CAD build for the part. Positions are in the model's coordinates, mm. A direction names the side the tool comes from. Coordinates: 2 decimals unless noted, no trailing zeros. Loops run counter-clockwise (first coordinate to the right, second up) from the corner with the lowest first, then second, coordinate; pieces in that order, holes last. Notation, with made-up numbers: (15.25, 20) -> (40.25, 20) arc R26 cw to (40.25, 48) -> close; hole circle Ø8 at (65, 57). An arc over 180 degrees is marked (long way). Write each question's results on one line, items separated by ' | '.
from build123d import *

# Parameters (mm, degrees)
SKETCH1_R           = 4
SKETCH1_R_2         = 1.625
BOSS_EXTRUDE2_DEPTH = 20
SKETCH2_R           = 4.9
BOSS_EXTRUDE3_DEPTH = 62
SKETCH6_R           = 1.625
CUT_EXTRUDE3_DEPTH  = 20


with BuildPart() as part:
    # Sketch1 → Boss-Extrude2 (new body)
    with BuildSketch(Plane(origin=(0, 0, 0), x_dir=(1, 0, 0), z_dir=(0, 1, 0))):
        Circle(SKETCH1_R)
        Circle(SKETCH1_R_2, mode=Mode.SUBTRACT)
    extrude(amount=BOSS_EXTRUDE2_DEPTH)

    # Sketch2 → Boss-Extrude3 (add)
    with BuildSketch(Plane.XZ):
        Circle(SKETCH2_R)
    extrude(amount=BOSS_EXTRUDE3_DEPTH)

    # Sketch6 → Cut-Extrude3 (cut)
    with BuildSketch(Plane.XZ.offset(62)):
        Circle(SKETCH6_R)
    extrude(amount=-CUT_EXTRUDE3_DEPTH, mode=Mode.SUBTRACT)


solid = part.part
1) Slice it at A-A (z = 0). Write the cut outline in (x, y) (3 decimals), then the cut area to 3 significant figures.
Outcome:
outline: (-4.9, -62) -> (-1.625, -62) -> (-1.625, -42) -> (1.625, -42) -> (1.625, -62) -> (4.9, -62) -> (4.9, 0) -> (4, 0) -> (4, 20) -> (1.625, 20) -> (1.625, 0) -> (-1.625, 0) -> (-1.625, 20) -> (-4, 20) -> (-4, 0) -> (-4.9, 0) -> close | area: 638 mm^2
2) Drill centre lines: L1, parallel to Z at x = 0, y = 8.5 (3 decimals); L2, parallel to Y at x = 4.5, z = 1.5. Where is each one in solid material? Low to high. Write a range as from..to.
Outcome:
L1: z = -4..-1.625, 1.625..4 | L2: y = -62..0
3) Which spindle directions (+Z, -Z, +X, -X, +Y, -Y) get a long thin tool onto all of the face, cutting with end or side? Do faces 4 (the cylindrical face through (-1.29, -52.14, -0.99)), 5 (the flat face through (2, 20, 0)), 6 (the cylindrical face through (-1.29, 9.86, 0.99)). Say none if no direction does.
Outcome:
face 4: -Y | face 5: +Z, -Z, +X, -X, +Y | face 6: +Y
4) Two-plate mould, pull along X, no slides. Class faces 1 (the cylindrical face through (-1.062, -30.566, -4.783)), 2 (the flat face through (2, -62, 0)), 3 (the flat face through (0, 0, 0)): pulls with the +X half, pulls with the -X half, needs draft (parallel to the pull), parting line crosses it, or undercut.
Outcome:
face 1: parting line crosses it | face 2: needs draft | face 3: undercut
5) Slice it at B-B (x = 0). Write the cut outline in (y, z) (3 decimals).
Outcome:
outline: (-62, -4.9) -> (0, -4.9) -> (0, -4) -> (20, -4) -> (20, -1.625) -> (0, -1.625) -> (0, 1.625) -> (20, 1.625) -> (20, 4) -> (0, 4) -> (0, 4.9) -> (-62, 4.9) -> (-62, 1.625) -> (-42, 1.625) -> (-42, -1.625) -> (-62, -1.625) -> close
6) Slice it at C-C (y = 4.5). Write the cut outline in (x, z) (3 decimals), then the cut area to 3 significant figures.
Outcome:
outline: circle Ø8 at (0, 0); hole circle Ø3.25 at (0, 0) | area: 42.0 mm^2
7) Pin check, flat tips, straight feed: pin 1 (3 mm diameter, centred on y = 4, z = -2, fed in from +X); pin 2 (3 mm diameter, centred on y = -35, z = -3.5, fed in from -X); pin 3 (1 mm diameter, centred on x = 0.5, z = 0.5, fed in from -Y). Stop position of each tip, or through.
Outcome:
pin 1: stops at x = 3.97 | pin 2: stops at x = -4.47 | pin 3: stops at y = -42
8) Slice it at D-D (y = -23.5). Write the cut outline in (x, z), then the cut area to 3 significant figures.
Outcome:
outline: circle Ø9.8 at (0, 0) | area: 75.4 mm^2
